Input: part model. Units: mm. Frame: model coordinates. Face numbers are marked on the shaded views. Give positions to 0.01 mm unless a question says otherwise; leave off trailing zeros. Loops run counter-clockwise (first coordinate to the right, second up) from the corner with the lowest first, then second, coordinate; pieces in that order, holes last. Notation, with made-up numbers: (-26, 78) -> (2, 78) arc R9 cw to (2, 82) -> close; hole circle Ø7 at (9.25, 89). An arc over 180 degrees is marked (long way). Answer as a JSON object with one key per item and string values.
Autodesk Inventor part; units mm, degrees
ref_plane "YZ Plane" through (0, 0, 0) normal (1, 0, 0) x (0, 1, 0)
ref_plane "XZ Plane" through (0, 0, 0) normal (0, 1, 0) x (-1, 0, 0)
ref_plane "XY Plane" through (0, 0, 0) normal (0, 0, 1) x (1, 0, 0)
sketch "Sketch1" plane through (0, 0, 0) normal (0, 1, 0) x (-1, 0, 0)
  line L0 (0, 0) -> (236.22, 0)
  line L1 (236.22, 0) -> (236.22, -375.92)
  line L2 (236.22, -375.92) -> (0, -375.92)
  line L3 (0, -375.92) -> (0, 0)
  dimension "d0" = 236.22
  dimension "d1" = 375.92
extrude "Extrusion1" add sketch "Sketch1" along normal blind 12.7
sketch "Sketch2" plane through (0, 12.7, 0) normal (0, 1, 0) x (1, 0, 0)
  line L0 (-236.22, 375.92) -> (-236.22, 0)
  line L1 (-236.22, 187.96) -> (-147.6375, 187.96)
  line L2 (0, 375.92) -> (-236.22, 375.92)
  line L3 (-147.6375, 375.92) -> (-147.6375, 275.92)
  line L4 (-236.22, 0) -> (0, 0)
  line L5 (-147.6375, 0) -> (-147.6375, 100)
  line L6 (-147.6375, 0) -> (-47.6375, 0) construction
  line L7 (-147.6375, 275.92) -> (-53.6575, 275.92)
  line L8 (-53.6575, 275.92) -> (-53.6575, 100)
  line L9 (-53.6575, 100) -> (-147.6375, 100)
  line L10 (-147.6375, 100) -> (-147.6375, 275.92)
  dimension "d4" = 88.5825
  dimension "d5" = 100
  dimension "d6" = 88.5825
  dimension "d7" = 100
  dimension "d8" = 90
  dimension "d9" = 88.5825
  dimension "d10" = 93.98
  dimension "d11" = 175.92
extrude "Extrusion2" add sketch "Sketch2" along normal blind 25.4 contours L10 L7 L8 L9
fillet "Fillet1" radius 4 4 edges at (-147.6375, 38.1, -187.96) (-53.6575, 38.1, -187.96) (-100.6475, 38.1, -100) (-100.6475, 38.1, -275.92)
sketch "Sketch3" plane through (0, 0, 0) normal (0, -1, 0) x (1, 0, 0)
  line L0 (0, -375.92) -> (0, 0)
  line L1 (-236.22, 0) -> (-236.22, -375.92)
  line L2 (0, 0) -> (-236.22, -375.92)
  line L3 (-236.22, -375.92) -> (-223.787, -356.1341)
  line L4 (0, 0) -> (-12.433, -19.7859)
  line L5 (-223.787, -356.1341) -> (-12.433, -356.1341)
  line L6 (-12.433, -356.1341) -> (-12.433, -19.7859)
  line L7 (-12.433, -19.7859) -> (-223.787, -19.7859)
  line L8 (-223.787, -19.7859) -> (-223.787, -356.1341)
  dimension "d15" = 23.368
  dimension "d16" = 23.368
extrude "Extrusion3" cut sketch "Sketch3" against normal blind 3
sketch "Sketch4" plane through (0, 38.1, 0) normal (0, 1, 0) x (1, 0, 0)
  circle A0 centre (-138.1475, 231.48) radius 1.75
  line L0 (-57.6575, 104) -> (-143.6375, 104)
  line L1 (-57.6575, 271.92) -> (-57.6575, 104)
  circle A1 centre (-63.1475, 231.48) radius 1.75
  circle A2 centre (-138.1475, 156.48) radius 1.75
  circle A3 centre (-63.1475, 156.48) radius 1.75
  point P0 (0, 0)
  dimension "d19" = 3.5
  dimension "d20" = 127.48
  dimension "d21" = 80.49
  dimension "d24" = 75
  dimension "d27" = 75
extrude "Extrusion4" cut sketch "Sketch4" against normal blind 3
properties part number "SpectreE165W_16in"
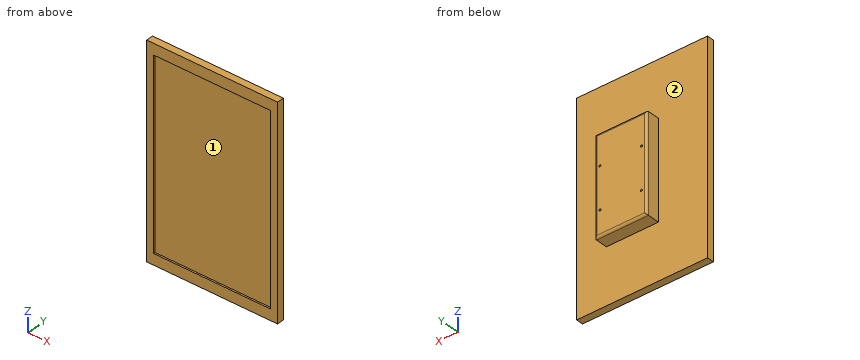
Q1. Section C-C, the plane y = 23. Return the cut outline in (x, z).
Evaluation:
{"outline": "(-147.64, -275.92) -> (-53.66, -275.92) -> (-53.66, -100) -> (-147.64, -100) -> close"}
Q2. Ray query, line 1 along X through (y, z) = (36.55, -156.48); line 2 along X through (y, z) = (34.5, -172.5); line 3 along Y through (x, z) = (-224.5, -151). Return the intervals inside material, ascending.
Evaluation:
{"line 1": "x = -146.8 to -139.9, -136.4 to -64.9, -61.4 to -54.5", "line 2": "x = -147.62 to -53.68", "line 3": "y = 0 to 12.7"}
Q3. Section B-B, the plane x = -152.5. Return the cut outline in (y, z), then the cut area to 3 significant figures.
Evaluation:
{"outline": "(0, -375.92) -> (12.7, -375.92) -> (12.7, 0) -> (0, 0) -> (0, -19.79) -> (3, -19.79) -> (3, -356.13) -> (0, -356.13) -> close", "area": "3,770 mm2"}
Q4. Draft query along Z for the marked faces 1 and 2. Return one class per face: +Z half, -Z half, draft (parallel to the pull), parting line (faces both ways), or undercut.
Evaluation:
{"face 1": "undercut", "face 2": "draft"}
Q5. Section A-A, the plane z = -26. Return the cut outline in (x, y), then the cut area to 3 significant figures.
Evaluation:
{"outline": "(-236.22, 0) -> (-223.79, 0) -> (-223.79, 3) -> (-12.43, 3) -> (-12.43, 0) -> (0, 0) -> (0, 12.7) -> (-236.22, 12.7) -> close", "area": "2,370 mm2"}
Q6. Pin query (flat end, axial travel): pin 1 (3 mm diameter, centred on x = -63.15, z = -156.48, fed in from -Y); pin 2 (1 mm diameter, centred on x = -62.5, z = -156, fed in from +Y); pin 3 (8 mm diameter, centred on x = -66.5, z = -90, fed in from +Y). Return the tip coordinate at first contact, or that it passes through.
Evaluation:
{"pin 1": "stops at y = 3", "pin 2": "stops at y = 35.1", "pin 3": "stops at y = 12.7"}
